```python
from build123d import *

# Parameters (mm, degrees)
SKETCH2_W          = 2
SKETCH2_H          = 0.3
SKETCH2_W_2        = 0.3
SKETCH2_H_2        = 2
CUT_EXTRUDE1_DEPTH = 0.5


with BuildPart() as part:
    # Sketch1 → Revolve1 (revolve)
    with BuildSketch(Plane.XY, mode=Mode.PRIVATE) as revolve1_sk:
        with BuildLine():
            Line((0, 0.8), (0, 0))
            Line((0, 0), (20, 0))
            Line((20, 0), (20, 0.5))
            Line((20, 0.5), (1, 0.5))
            Line((1, 0.5), (1, 0.8))
            ThreePointArc((1, 0.8), (0.941421356, 0.941421356), (0.8, 1))
            Line((0.8, 1), (0.2, 1))
            ThreePointArc((0.2, 1), (0.058578644, 0.941421356), (0, 0.8))
        make_face()
    revolve(revolve1_sk.sketch.rotate(Axis((0, 0, 0), (1, 0, 0)), 90), axis=Axis((0, 0, 0), (1, 0, 0)))

    # Sketch2 → Cut-Extrude1 (cut)
    with BuildSketch(Plane.ZY):
        Rectangle(SKETCH2_W, SKETCH2_H)
        Rectangle(SKETCH2_W_2, SKETCH2_H_2)
    extrude(amount=-CUT_EXTRUDE1_DEPTH, mode=Mode.SUBTRACT)


solid = part.part
```
Design review of the part built by this model. Coordinates are the model's own, in mm. Coordinates: 2 decimals unless noted, no trailing zeros. Loops run counter-clockwise (first coordinate to the right, second up) from the corner with the lowest first, then second, coordinate; pieces in that order, holes last. Notation, with made-up numbers: (68.5, 5.25) - (109.5, 5.25) arc R26 cw to (109.5, 40.25) - close; hole circle Ø10 at (35, 70). An arc over 180 degrees is marked (long way). Use CSV: the item, a comma, the result in double quotes. Start each with the question number.
1) For pin 1 Ø0.6 at (x, y) = (0.5, -0.5) entering from -Z; pin 2 Ø1 at (x, y) = (4.5, 0.5) entering from +Z, all flat-tipped, find the tip position at first contact; note any pin that passes through.
2) The part is to be moulded in two halves that separate along Z. For faces 1 (the flat face through (0.5, 0, 0)), 2 (the cylindrical face through (0.5, 0.89, 0.46)), 3 (the flat face through (20, 0, 0)), say which applies: +Z half, -Z half, draft (parallel to the pull), parting line (faces both ways), or undercut.
3) Wall thickness on L1, parallel to X at y = -0.25, z = -0.6; L2, parallel to Y at x = 16.5, z = -0.05; L3, parallel to X at y = -0.45, z = -0.1: over which ranges is each line inside the solid? List them lowest first. Write a range as from..to.
4) Consider section A-A on x = 13. Write out the cut boundary in (y, z), then the cut area to 3 significant figures.
Geometry says:
1,pin 1,"z = -0.98"
1,pin 2,"z = 0.5"
2,face 1,"undercut"
2,face 2,"parting line"
2,face 3,"draft"
3,L1,"0..1"
3,L2,"-0.5..0.5"
3,L3,"0.5..20"
4,outline,"circle Ø1 at (0, 0)"
4,area,"0.785 mm^2"
